Read the model definition and answer for the solid it produces. Units are mm, in the model's axes. A direction names the side the tool comes from. Round coordinates to 2 decimals unless told otherwise and drop trailing zeros. Order: outer loops, then holes, each group sorted by start corner. A loop starts at its lowest first (then second) coordinate and runs counter-clockwise, first axis right, second up. Notation, with made-up numbers: (33, -28.5) - (76, -28.5) arc R23 cw to (76, -18.5) - close; hole circle Ø1 at (-21, 64.25). An arc over 180 degrees is marked (long way). Answer as a JSON object with one key per item and string values. Group by question number.
Q1. Given pin 1 Ø10 at (x, y) = (-11.5, 46.5) entering from +Z; pin 2 Ø0.8 at (x, y) = (-7, 58.5) entering from -Z; pin 3 Ø24.5 at (y, z) = (41.5, 45) entering from -X; pin 4 Ø1.7 at (x, z) = (0, 44.1) entering from +Y, each flat-ended and moving along its own axis, determine where each tip first touches the part or whether it passes through.
Q2. The mould has two halves that part along Y. Classify faces 1 (the flat face through (0, 44, 60.878)), 2 (the cylindrical face through (30.998, -31.037, 38.633)), 3 (the cylindrical face through (-18.1, 18.14, 38.63)), 4 (the flat face through (0, -19.05, 38)): pulls with the +Y half, pulls with the -Y half, needs draft (parallel to the pull), parting line crosses it, or undercut.
Q3. Consider line 1 (X direction, y = 6, z = 33); line 2 (Y direction, x = -25, z = 47); line 3 (Y direction, x = 25, z = 58). Determine where each line is inside the solid, lowest interval first.
Q4. A cutting plane is placed at B-B on x = 0. Count the separate pieces of the cut face and the enclosed holes in it, and give its area (3 significant figures).
Q5. A cutting plane is placed at A-A on y = 25.4. Determine the outline of the cut face in (x, z).
Q6. A cutting plane is placed at D-D on y = 46. Determine the outline of the cut face in (x, z), and give its area (3 significant figures).
Q7. A tool of negligible diameter and unlimited length cuts with its end or side. For faces 5 (the cylindrical face through (0.18, 37.96, 34.09)), 6 (the flat face through (0, 44, 10.078)), 7 (the flat face through (-28.514, 43, 36)), from which of +Z, -Z, +X, -X, +Y, -Y can it reach the whole face along a straight path? Write none if from no direction.
```python
from build123d import *

# Parameters (mm, degrees)
SKETCH1_W                = 63.5
SKETCH1_H                = 63.5
BOSS_EXTRUDE1_DEPTH      = 76.2
M5_CLEARANCE_HOLE1_D     = 5.5
SKETCH4_W                = 38.1
SKETCH4_H                = 38.1
CUT_EXTRUDE1_DEPTH       = 89.44526556
FILLET1_R                = 2.5
FILLET2_R                = 3.175
SKETCH5_W                = 57.027431562
SKETCH5_H                = 50.8
BOSS_EXTRUDE2_DEPTH      = 27.178
SKETCH7_W                = 38.354
SKETCH7_H                = 8.128
CUT_EXTRUDE2_DEPTH       = 1.524
M3_CLEARANCE_HOLE1_D     = 2.8
M3_CLEARANCE_HOLE1_DEPTH = 38.354
FILLET3_SIZE             = 5
FILLET4_SIZE             = 2
FILLET5_SIZE             = 2


with BuildPart() as part:
    # Sketch1 → Boss-Extrude1 (new body)
    with BuildSketch(Plane.XY):
        Rectangle(SKETCH1_W, SKETCH1_H)
    extrude(amount=BOSS_EXTRUDE1_DEPTH)

    # M5 Clearance Hole1 (through all)
    with Locations(Plane.XY.offset(76.2)):
        with Locations((25.4, -25.4), (25.4, 25.4), (-25.4, -25.4), (-25.4, 25.4)):
            Hole(M5_CLEARANCE_HOLE1_D / 2)

    # Sketch4 → Cut-Extrude1 (cut, through all)
    with BuildSketch(Plane(origin=(0, 0, 0), x_dir=(-1, 0, 0), z_dir=(0, 0, -1))):
        Rectangle(SKETCH4_W, SKETCH4_H)
    extrude(amount=-CUT_EXTRUDE1_DEPTH, mode=Mode.SUBTRACT)

    # Fillet1
    fillet1_edges = [part.edges().sort_by_distance(p)[0] for p in [
        (31.75, -31.75, 38.1),
        (-31.75, -31.75, 38.1),
        (-31.75, 31.75, 38.1),
        (31.75, 31.75, 38.1),
    ]]
    fillet(fillet1_edges, radius=FILLET1_R)

    # Fillet2
    fillet2_edges = [part.edges().sort_by_distance(p)[0] for p in [
        (19.05, -19.05, 38.1),
        (19.05, 19.05, 38.1),
        (-19.05, 19.05, 38.1),
        (-19.05, -19.05, 38.1),
    ]]
    fillet(fillet2_edges, radius=FILLET2_R)

    # Sketch5 → Boss-Extrude2 (add)
    with BuildSketch(Plane(origin=(0, 31.75, 0), x_dir=(1, 0, 0), z_dir=(0, 1, 0))):
        with Locations((0, -35.47764662)):
            Rectangle(SKETCH5_W, SKETCH5_H)
    extrude(amount=BOSS_EXTRUDE2_DEPTH)

    # Sketch7 → Cut-Extrude2 (cut)
    with BuildSketch(Plane(origin=(0, 58.928, 0), x_dir=(1, 0, 0), z_dir=(0, 1, 0))):
        with Locations((-274.796433557, 103.138535486)):
            Rectangle(SKETCH7_W, SKETCH7_H)
        with Locations((0, -35.47764662)):
            Rectangle(SKETCH7_W, SKETCH7_H)
        with Locations((0, -44.101274776)):
            Rectangle(SKETCH7_W, SKETCH7_H)
    extrude(amount=-CUT_EXTRUDE2_DEPTH, mode=Mode.SUBTRACT)

    # M3 Clearance Hole1
    with Locations(Plane(origin=(0, 57.404, 0), x_dir=(1, 0, 0), z_dir=(0, 1, 0))):
        with Locations((0, -44.101274776), (0, -35.47764662)):
            Hole(M3_CLEARANCE_HOLE1_D / 2, depth=M3_CLEARANCE_HOLE1_DEPTH)

    # Fillet3
    # a fillet whose section is not a circle: 5 mm, written as the material it takes off along each edge
    with BuildSketch(Plane(origin=(-41.013715781, 58.928, 10.07764662), x_dir=(0, -1, 0), z_dir=(1, 0, 0)), Plane(origin=(41.013715781, 58.928, 60.87764662), x_dir=(0, -1, 0), z_dir=(-1, 0, 0))) as fillet3_piece_1:
        with BuildLine():
            Bezier((FILLET3_SIZE, 0), (0, 0), (0, -FILLET3_SIZE), weights=[1, 1, 1])
            Line((0, -FILLET3_SIZE), (0, 0))
            Line((0, 0), (FILLET3_SIZE, 0))
        make_face()
    extrude(amount=82.027431561, mode=Mode.SUBTRACT)
    with BuildSketch(Plane(origin=(28.513715781, 58.928, -2.42235338), x_dir=(0, -1, 0), z_dir=(0, 0, 1)), Plane(origin=(-28.513715781, 58.928, 73.37764662), x_dir=(0, -1, 0), z_dir=(0, 0, -1))) as fillet3_piece_2:
        with BuildLine():
            Bezier((FILLET3_SIZE, 0), (0, 0), (0, -FILLET3_SIZE), weights=[1, 1, 1])
            Line((0, -FILLET3_SIZE), (0, 0))
            Line((0, 0), (FILLET3_SIZE, 0))
        make_face()
    extrude(amount=75.8, mode=Mode.SUBTRACT)

    # Fillet4
    # a fillet whose section is not a circle: 2 mm, written as the material it adds along each edge
    with BuildSketch(Plane(origin=(28.513715781, 31.75, 60.87764662), x_dir=(0, 0, 1), z_dir=(-1, 0, 0))) as fillet4_piece_1:
        with BuildLine():
            Bezier((FILLET4_SIZE, 0), (0, 0), (0, FILLET4_SIZE), weights=[1, 1, 1])
            Line((0, FILLET4_SIZE), (0, 0))
            Line((0, 0), (FILLET4_SIZE, 0))
        make_face()
    extrude(amount=57.027431561)

    # Fillet5
    # a fillet whose section is not a circle: 2 mm, written as the material it adds along each edge
    with BuildSketch(Plane(origin=(-28.513715781, 31.75, 10.07764662), x_dir=(0, 1, 0), z_dir=(1, 0, 0))) as fillet5_piece_1:
        with BuildLine():
            Bezier((FILLET5_SIZE, 0), (0, 0), (0, -FILLET5_SIZE), weights=[1, 1, 1])
            Line((0, -FILLET5_SIZE), (0, 0))
            Line((0, 0), (FILLET5_SIZE, 0))
        make_face()
    extrude(amount=57.027431561)


solid = part.part
```
Result set:
{
 "1": {"pin 1": "stops at z = 60.88", "pin 2": "stops at z = 11.84", "pin 3": "stops at x = -31.75", "pin 4": "stops at y = -19.05"},
 "2": {"face 1": "needs draft", "face 2": "pulls with the -Y half", "face 3": "undercut", "face 4": "undercut"},
 "3": {"line 1": "x = -31.75 to -19.05, 19.05 to 31.75", "line 2": "y = -31.75 to -28.12, -22.68 to 22.68, 28.12 to 58.8", "line 3": "y = -31.75 to -28.12, -22.68 to 22.68, 28.12 to 58.64"},
 "4": {"separate pieces": "4", "enclosed holes": "0", "area": "3,070 mm²"},
 "5": {"outline": "(-31.75, 0) - (-28.15, 0) - (-28.15, 76.2) - (-31.75, 76.2) - close; (-22.65, 0) - (22.65, 0) - (22.65, 76.2) - (-22.65, 76.2) - close; (28.15, 0) - (31.75, 0) - (31.75, 76.2) - (28.15, 76.2) - close; hole circle Ø2.8 at (0, 35.48); hole circle Ø2.8 at (0, 44.1)"},
 "6": {"outline": "(-28.51, 10.08) - (28.51, 10.08) - (28.51, 60.88) - (-28.51, 60.88) - close; hole circle Ø2.8 at (0, 35.48); hole circle Ø2.8 at (0, 44.1)", "area": "2,880 mm²"},
 "7": {"face 5": "+Y", "face 6": "-Z, +X, -X, +Y", "face 7": "+Z, -Z, -X, +Y"}
}
